from build123d import *

# Parameters (mm, degrees)
EXTRUDE_1_DEPTH     = 1
CUT_EXTRUDE_4_DEPTH = 54.935146241
SKETCH_4_R          = 1.5
CUT_EXTRUDE_5_DEPTH = 54.935146241
CUT_EXTRUDE1_START  = -1
CUT_EXTRUDE1_DEPTH  = 1
SKETCH4_W           = 98
SKETCH4_H           = 10
BOSS_EXTRUDE1_DEPTH = 1


with BuildPart() as part:
    # Эскиз1 → Бобышка-Вытянуть1 (new body)
    with BuildSketch(Plane.XY):
        Polygon((-49, 5.839183832), (-49, -22.516660498), (49, -22.516660498), (49, 5.839183832), (49, 15.839183832), (-49, 15.839183832), align=None)
    extrude(amount=EXTRUDE_1_DEPTH)

    # Эскиз2 → Вырез-Вытянуть4 (cut, through all)
    with BuildSketch(Plane(origin=(0, 0, 0), x_dir=(-1, 0, 0), z_dir=(0, 0, -1))):
        with BuildLine():
            Line((27.226146034, -9.122134253), (15.739905482, -9.122134253))
            ThreePointArc((15.739905482, -9.122134253), (15.10500819, -9.461530461), (14.917793913, -10.156681647))
            Line((14.917793913, -10.156681647), (17.442090319, -18.930924047))
            ThreePointArc((17.442090319, -18.930924047), (18.050493328, -19.909298147), (19.122649731, -20.331021695))
            Line((19.122649731, -20.331021695), (30.826843589, -20.331021695))
            ThreePointArc((30.826843589, -20.331021695), (31.459345435, -19.990005133), (31.64325008, -19.295361367))
            Line((31.64325008, -19.295361367), (29.100959308, -10.488607797))
            ThreePointArc((29.100959308, -10.488607797), (28.40806584, -9.469896887), (27.226146034, -9.122134253))
        make_face()
        with BuildLine():
            Line((-31.64325008, -19.295361367), (-29.100959308, -10.488607797))
            ThreePointArc((-29.100959308, -10.488607797), (-28.40806584, -9.469896887), (-27.226146034, -9.122134253))
            Line((-27.226146034, -9.122134253), (-15.739905482, -9.122134253))
            ThreePointArc((-15.739905482, -9.122134253), (-15.10500819, -9.461530461), (-14.917793913, -10.156681647))
            Line((-14.917793913, -10.156681647), (-17.442090319, -18.930924047))
            ThreePointArc((-17.442090319, -18.930924047), (-18.050493328, -19.909298147), (-19.122649731, -20.331021695))
            Line((-19.122649731, -20.331021695), (-30.826843589, -20.331021695))
            ThreePointArc((-30.826843589, -20.331021695), (-31.459345435, -19.990005133), (-31.64325008, -19.295361367))
        make_face()
    extrude(amount=-CUT_EXTRUDE_4_DEPTH, mode=Mode.SUBTRACT)

    # Эскиз4 → Вырез-Вытянуть5 (cut, through all)
    with BuildSketch(Plane(origin=(0, 0, 0), x_dir=(-1, 0, 0), z_dir=(0, 0, -1))):
        with Locations((36, -7.524952718)):
            Circle(SKETCH_4_R)
        with Locations((-36, -7.524952718)):
            Circle(SKETCH_4_R)
    extrude(amount=-CUT_EXTRUDE_5_DEPTH, mode=Mode.SUBTRACT)

    # Sketch3 → Cut-Extrude1 (cut)
    with BuildSketch(Plane.XY.offset(1).offset(CUT_EXTRUDE1_START)):
        with BuildLine():
            Line((8.652344227, -7.068131311), (12.085677561, -18.961546856))
            add(Edge.make_bspline(
                [(12.085677561, -18.961546856), (12.485677561, -20.347187502), (13.871318207, -20.347187502)],
                knots=[0.857071948, 0.857071948, 0.857071948, 2.427868275, 2.427868275, 2.427868275], degree=2, weights=[1, 0.707106781, 1]))
            Line((13.871318207, -20.347187502), (32.461996875, -20.347187502))
            add(Edge.make_bspline(
                [(32.461996875, -20.347187502), (33.393769403, -20.347187502), (33.496157418, -19.484255682)],
                knots=[2.427868275, 2.427868275, 2.427868275, 3.611858299, 3.611858299, 3.611858299], degree=2, weights=[1, 0.829829079, 1]))
            add(Edge.make_bspline(
                [(33.496157418, -19.484255682), (33.529743577, -19.201189685), (33.607326061, -18.923570429), (33.853252735, -18.417152493), (34.025349409, -18.183932413), (34.436238564, -17.8036127), (34.681879478, -17.649935655), (35.200024528, -17.435065661), (35.479061866, -17.369439067), (35.76148791, -17.34207634)],
                knots=[0, 0, 0, 0, 0.25, 0.25, 0.5, 0.5, 0.75, 0.75, 1, 1, 1, 1], degree=3))
            add(Edge.make_bspline(
                [(35.76148791, -17.34207634), (36.181169226, -17.301415694), (36.592378309, -17.212108423), (37.170380488, -16.959028015), (37.354968395, -16.854344533), (37.687544868, -16.599797528), (37.83830967, -16.446579579), (38.076557482, -16.101495837), (38.166209489, -15.905573827), (38.271501218, -15.499696694), (38.288800836, -15.285469364), (38.263278752, -14.867475934), (38.220734772, -14.657932914), (38.094284502, -14.258193956), (38.010543981, -14.065974434), (37.910619322, -13.879789794)],
                knots=[0, 0, 0, 0, 0.25, 0.25, 0.375, 0.375, 0.5, 0.5, 0.625, 0.625, 0.75, 0.75, 0.875, 0.875, 1, 1, 1, 1], degree=3))
            Line((37.910619322, -13.879789794), (35.170885606, -8.774980446))
            ThreePointArc((35.170885606, -8.774980446), (34.803783463, -8.429975368), (34.571610551, -7.982886756))
            ThreePointArc((34.571610551, -7.982886756), (34.527886571, -7.812845152), (34.504331156, -7.638859302))
            add(Edge.make_bspline(
                [(34.504331156, -7.638859302), (33.03670289, -5.782259548), (30.630891119, -5.783194379)],
                knots=[4.00651056, 4.00651056, 4.00651056, 5.38030343, 5.38030343, 5.38030343], degree=2, weights=[1, 0.773217832, 1]))
            Line((30.630891119, -5.783194379), (28.778313515, -5.783914238))
            add(Edge.make_bspline(
                [(28.778313515, -5.783914238), (28.498733332, -5.682490665), (28.228663541, -5.682490665)],
                knots=[5.18447533, 5.18447533, 5.18447533, 5.569460928, 5.569460928, 5.569460928], degree=2, weights=[1, 0.981530397, 1]))
            Line((28.228663541, -5.682490665), (9.637984874, -5.682490665))
            add(Edge.make_bspline(
                [(9.637984874, -5.682490665), (8.252344227, -5.682490665), (8.652344227, -7.068131311)],
                knots=[5.569460928, 5.569460928, 5.569460928, 7.140257255, 7.140257255, 7.140257255], degree=2, weights=[1, 0.707106781, 1]))
        make_face()
        with BuildLine():
            Line((-35.170885606, -8.774980446), (-37.925052204, -13.906681863))
            add(Edge.make_bspline(
                [(-37.925052204, -13.906681863), (-38.025225081, -14.093328995), (-38.109806595, -14.28778394), (-38.235924368, -14.687324932), (-38.278394681, -14.895918794), (-38.297414091, -15.212202185), (-38.296322734, -15.317469634), (-38.277441195, -15.527644209), (-38.259343447, -15.633280004), (-38.205994928, -15.836909506), (-38.170798519, -15.935630825), (-38.082894213, -16.126717018), (-38.029532599, -16.219817403), (-37.849055501, -16.479499021), (-37.698892817, -16.631115336), (-37.362837335, -16.886481906), (-37.179664999, -16.989484869), (-36.595923377, -17.242719775), (-36.186794345, -17.329699001), (-35.766265682, -17.369273893)],
                knots=[0, 0, 0, 0, 0.125, 0.125, 0.25, 0.25, 0.3125, 0.3125, 0.375, 0.375, 0.4375, 0.4375, 0.5, 0.5, 0.625, 0.625, 0.75, 0.75, 1, 1, 1, 1], degree=3))
            add(Edge.make_bspline(
                [(-33.495182661, -19.492227082), (-33.738478544, -17.560103824), (-35.766265682, -17.369273893)],
                knots=[5.81913938, 5.81913938, 5.81913938, 6.905546226, 6.905546226, 6.905546226], degree=2, weights=[1, 0.856057288, 1]))
            add(Edge.make_bspline(
                [(-33.495182661, -19.492227082), (-33.387524752, -20.347187502), (-32.461996875, -20.347187502)],
                knots=[2.677546726, 2.677546726, 2.677546726, 3.855317033, 3.855317033, 3.855317033], degree=2, weights=[1, 0.83156042, 1]))
            Line((-32.461996875, -20.347187502), (-13.871318207, -20.347187502))
            add(Edge.make_bspline(
                [(-13.871318207, -20.347187502), (-12.46794332, -20.347187502), (-12.080702928, -18.943926093)],
                knots=[3.855317033, 3.855317033, 3.855317033, 5.438830393, 5.438830393, 5.438830393], degree=2, weights=[1, 0.702596367, 1]))
            Line((-12.080702928, -18.943926093), (-8.83075434, -7.166932971))
            add(Edge.make_bspline(
                [(-8.83075434, -7.166932971), (-8.45309236, -5.798381309), (-9.82190813, -5.798913193)],
                knots=[5.438830393, 5.438830393, 5.438830393, 6.997298301, 6.997298301, 6.997298301], degree=2, weights=[1, 0.711452073, 1]))
            Line((-9.82190813, -5.798913193), (-30.645016113, -5.807004464))
            add(Edge.make_bspline(
                [(-30.645016113, -5.807004464), (-33.032902471, -5.807932329), (-34.505069218, -7.648167801)],
                knots=[0.90305787, 0.90305787, 0.90305787, 2.269113721, 2.269113721, 2.269113721], degree=2, weights=[1, 0.775665219, 1]))
            ThreePointArc((-34.505069218, -7.648167801), (-34.53118454, -7.829224215), (-34.579145022, -8.005755309))
            ThreePointArc((-34.579145022, -8.005755309), (-34.811085633, -8.43954696), (-35.170885606, -8.774980446))
        make_face()
    extrude(amount=CUT_EXTRUDE1_DEPTH, mode=Mode.SUBTRACT)

    # Sketch4 → Boss-Extrude1 (add)
    with BuildSketch(Plane.XY.offset(1)):
        with Locations((0, -27.516660498)):
            Rectangle(SKETCH4_W, SKETCH4_H)
    extrude(amount=-BOSS_EXTRUDE1_DEPTH)


solid = part.part
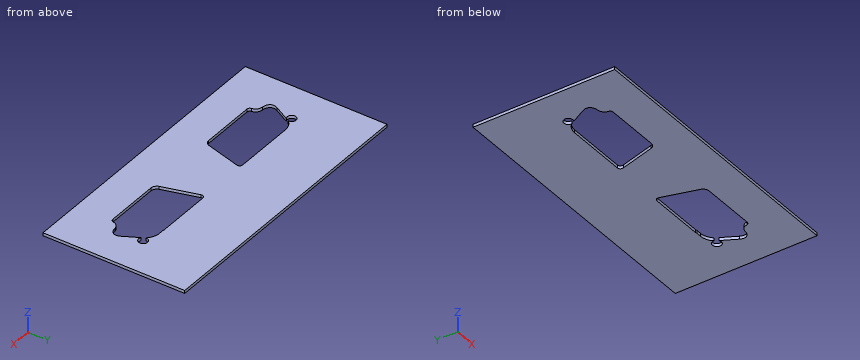
Read the model definition and answer for the solid it produces. Units are mm, in the model's axes. Coordinates: 2 decimals unless noted, no trailing zeros. Loops run counter-clockwise (first coordinate to the right, second up) from the corner with the lowest first, then second, coordinate; pieces in that order, holes last. Notation, with made-up numbers: (31, -35.5) -> (68, -35.5) arc R22 ccw to (68, -14.5) -> close; hole circle Ø7 at (17, 87). An arc over 180 degrees is marked (long way). Write item = value, one per line. Start each with the question number.
1) Given P1, Ø2.5, axis at x = -36, y = -7.52, coming from the -Z side, flat-ended and moving along its own axis, determine where the tip first touches the part or whether it passes through.
2) Find the intervals of material crossed by L1, parallel to Y at x = -14, z = 0.45; L2, parallel to Y at x = 19.5, z = 0.9; L3, parallel to Y at x = 36, z = 0.6, in increasing order. Write a range as from..to.
3) The part is cut by section B-B, the plane z = 0.5. State how many separate pieces and enclosed holes the cut face has, plus the area to 3 significant figures.
4) The part is cut by section C-C, the plane x = -21. Determine the outline of the cut face in (y, z).
5) The part is cut by section A-A, the plane x = 21. Determine the outline of the cut face in (y, z), plus the area to 3 significant figures.
Result:
q1.P1 = through
q2.L1 = -32.52..-20.35, -5.8..15.84
q2.L2 = -32.52..-20.35, -5.68..15.84
q2.L3 = -32.52..-17.31, -10.32..-9.02, -6.02..15.84
q3.separate_pieces = 1
q3.enclosed_holes = 2
q3.area = 3,990 mm²
q4.outline = (-32.52, 0) -> (-20.35, 0) -> (-20.35, 1) -> (-32.52, 1) -> close; (-5.8, 0) -> (15.84, 0) -> (15.84, 1) -> (-5.8, 1) -> close
q5.outline = (-32.52, 0) -> (-20.35, 0) -> (-20.35, 1) -> (-32.52, 1) -> close; (-5.68, 0) -> (15.84, 0) -> (15.84, 1) -> (-5.68, 1) -> close
q5.area = 33.7 mm²
